The listing builds one solid part. Answer for the finished solid, in the listing's coordinates (mm). A direction names the side the tool comes from. Round coordinates to 2 decimals unless told otherwise and drop trailing zeros. Write each loop counter-clockwise with the first axis right and the second up, starting at its lowest first coordinate (ties: lowest second). Pieces come first, ordered by that corner, then holes.
(1) The mould has two halves that part along X. Classify faces 1 (the face through (53.461, 15.304, -6.346)), 2 (the face through (90, 21, -37)), 3 (the face through (65, 21, -15)), 4 (the face through (77, 41.5, -15)): +X half, -X half, draft (parallel to the pull), parting line (faces both ways), or undercut.
(2) A cutting plane is placed at B-B, the plane z = -47. Give the vertices of the cut face in (x, y).
(3) Find the intervals of material crossed by probe 1 along X at (y, z) = (1.15, -3); probe 2 along Z at (x, y) = (3, 0.8); probe 3 along Z at (x, y) = (89, 28), in increasing order.
(4) Each of these flat-tipped pins is pushed along its axis until it touches: pin 1 Ø2 at (x, z) = (50, -27.5) entering from +Y; pin 2 Ø8 at (x, y) = (60, 6.5) entering from +Z; pin 3 Ø8 at (y, z) = (17.5, -36) entering from -X; pin 4 Ø3.5 at (x, z) = (3, -47) entering from -Y. Where does it stop, or does it pass through?
(5) A cutting plane is placed at D-D, the plane x = 71. Give the vertices of the cut face in (y, z), and give its area (3 significant figures).
(6) A cutting plane is placed at C-C, the plane y = 33.5. Give the vertices of the cut face in (x, z), and give its area (3 significant figures).
(7) For faces 5 (the face through (50, 29.5, -37)), 6 (the face through (77, 21, -10)), 7 (the face through (77, 21, -20)), 8 (the face through (65, 21, -37)), determine the directions among +Z, -Z, +X, -X, +Y, -Y from which every point of the face is accessible in a straight line to the end or side of a thin tool.
(8) A cutting plane is placed at A-A, the plane y = 21.5. Give the vertices of the cut face in (x, z), and give its area (3 significant figures).
from build123d import *

# Parameters (mm, degrees)
ESBO_O1_W                = 110
ESBO_O1_H                = 50
RESSALTO_EXTRUS_O1_DEPTH = 1.5
ESBO_O2_R                = 2
CORTE_EXTRUS_O1_DEPTH    = 1.5
ESBO_O4_R                = 7.5
ESBO_O4_W                = 25
ESBO_O4_H                = 10
RESSALTO_EXTRUS_O3_DEPTH = 40
ESBO_O5_W                = 39
ESBO_O5_H                = 12
CORTE_EXTRUS_O2_DEPTH    = 60


with BuildPart() as part:
    # Esboço1 → Ressalto-extrusão1 (new body)
    with BuildSketch(Plane(origin=(0, 0, 0), x_dir=(1, 0, 0), z_dir=(0, 1, 0))):
        with Locations((55, 25)):
            Rectangle(ESBO_O1_W, ESBO_O1_H)
    extrude(amount=RESSALTO_EXTRUS_O1_DEPTH)

    # Esboço2 → Corte-extrusão1 (cut)
    with BuildSketch(Plane(origin=(0, 1.5, 0), x_dir=(1, 0, 0), z_dir=(0, 1, 0))):
        with Locations((107, 3)):
            Circle(ESBO_O2_R)
        with Locations((107, 47)):
            Circle(ESBO_O2_R)
        with Locations((3, 3)):
            Circle(ESBO_O2_R)
        with Locations((3, 47)):
            Circle(ESBO_O2_R)
    extrude(amount=-CORTE_EXTRUS_O1_DEPTH, mode=Mode.SUBTRACT)

    # Esboço4 → Ressalto-extrusão3 (add)
    with BuildSketch(Plane(origin=(0, 1.5, 0), x_dir=(1, 0, 0), z_dir=(0, 1, 0))):
        with Locations((50, 37)):
            Circle(ESBO_O4_R)
        with Locations((50, 13)):
            Circle(ESBO_O4_R)
        with Locations((77.5, 37)):
            Rectangle(ESBO_O4_W, ESBO_O4_H)
        with Locations((77.5, 15)):
            Rectangle(ESBO_O4_W, ESBO_O4_H)
    extrude(amount=RESSALTO_EXTRUS_O3_DEPTH)

    # Esboço5 → Corte-extrusão2 (cut)
    with BuildSketch(Plane(origin=(0, 0, 0), x_dir=(0, 0, -1), z_dir=(1, 0, 0))):
        with Locations((25, 35.5)):
            Rectangle(ESBO_O5_W, ESBO_O5_H)
    extrude(amount=CORTE_EXTRUS_O2_DEPTH, mode=Mode.SUBTRACT)


solid = part.part
Solutions:
1. face 1: undercut
1. face 2: +X half
1. face 3: undercut
1. face 4: draft
2. outline: (0, 0) - (1, 0) - (1, 1.5) - (0, 1.5) - close; (5, 0) - (105, 0) - (105, 1.5) - (5, 1.5) - close; (109, 0) - (110, 0) - (110, 1.5) - (109, 1.5) - close
3. probe 1: x = 0 to 1, 5 to 105, 109 to 110
3. probe 2: z = -50 to -49, -45 to -5, -1 to 0
3. probe 3: z = -42 to -32, -20 to -10
4. pin 1: stops at y = 1.5
4. pin 2: stops at z = -8.5
4. pin 3: stops at x = 42.5
4. pin 4: passes through
5. outline: (0, -50) - (1.5, -50) - (1.5, -42) - (41.5, -42) - (41.5, -32) - (1.5, -32) - (1.5, -20) - (41.5, -20) - (41.5, -10) - (1.5, -10) - (1.5, 0) - (0, 0) - close
5. area: 875 mm2
6. outline: (65, -42) - (90, -42) - (90, -32) - (65, -32) - close; (65, -20) - (90, -20) - (90, -10) - (65, -10) - close
6. area: 500 mm2
7. face 5: +Z, -Z, -X, +Y
7. face 6: +Z, +X, +Y
7. face 7: +X, +Y
7. face 8: +Z, -Z, +Y
8. outline: circle Ø15 at (50, -37); circle Ø15 at (50, -13); (65, -42) - (90, -42) - (90, -32) - (65, -32) - close; (65, -20) - (90, -20) - (90, -10) - (65, -10) - close
8. area: 853 mm2
